The listing builds one solid part. Answer for the finished solid, in the listing's coordinates (mm). A direction names the side the tool comes from. Coordinates: 2 decimals unless noted, no trailing zeros. Write each loop counter-clockwise with the first axis right and the second up, starting at its lowest first coordinate (ties: lowest second). Pieces come first, ordered by that corner, then holes.
from build123d import *

# Parameters (mm, degrees)
SKETCH_1_R      = 2.5
SKETCH_1_R_2    = 4.5
SKETCH_1_R_3    = 3
SKETCH_1_R_4    = 1.5
EXTRUDE_1_DEPTH = 2.5


with BuildPart() as part:
    # Эскиз1 → Бобышка-Вытянуть1 (new, symmetric)
    # profile 1 of 7: a face of its own
    with BuildSketch(Plane.XY):
        with BuildLine():
            ThreePointArc((-0.9, -4.409081537), (-4.5, 0), (-0.9, 4.409081537))
            Line((-0.9, 4.409081537), (-10.5, 2.449489743))
            ThreePointArc((-10.5, 2.449489743), (-8.41886117, 1.936491673), (-7.5, 0))
            ThreePointArc((-7.5, 0), (-8.41886117, -1.936491673), (-10.5, -2.449489743))
            Line((-10.5, -2.449489743), (-0.9, -4.409081537))
        make_face()
    # profile 2 of 7: a face of its own
    with BuildSketch(Plane.XY):
        with Locations((-10, 0)):
            Circle(SKETCH_1_R)
    # profile 3 of 7: a face of its own
    with BuildSketch(Plane.XY):
        Circle(SKETCH_1_R_2)
        Circle(SKETCH_1_R, mode=Mode.SUBTRACT)
    # profile 4 of 7: a face of its own
    with BuildSketch(Plane.XY):
        with BuildLine():
            Line((12.375, 2.976470225), (0.5625, 4.464705337))
            ThreePointArc((0.5625, 4.464705337), (3.375, 2.976470225), (4.5, 0))
            ThreePointArc((4.5, 0), (3.375, -2.976470225), (0.5625, -4.464705337))
            Line((0.5625, -4.464705337), (12.375, -2.976470225))
            ThreePointArc((12.375, -2.976470225), (9, 0), (12.375, 2.976470225))
        make_face()
    # profile 5 of 7: a face of its own
    with BuildSketch(Plane.XY):
        with Locations((12, 0)):
            Circle(SKETCH_1_R_3)
        with Locations((12, 0)):
            Circle(SKETCH_1_R_4, mode=Mode.SUBTRACT)
    # profile 6 of 7: a face of its own
    with BuildSketch(Plane.XY):
        with BuildLine():
            Line((-1.5, -2), (-1.5, 2))
            ThreePointArc((-1.5, 2), (-2.5, 0), (-1.5, -2))
        make_face()
    # profile 7 of 7: a face of its own
    with BuildSketch(Plane.XY):
        with BuildLine():
            ThreePointArc((2.5, 0), (2.236067977, 1.118033989), (1.5, 2))
            Line((1.5, 2), (1.5, -2))
            ThreePointArc((1.5, -2), (2.236067977, -1.118033989), (2.5, 0))
        make_face()
    extrude(amount=EXTRUDE_1_DEPTH, both=True)


solid = part.part
1. Find the intervals of material crossed by L1, parallel to X at y = -1, z = -1.9; L2, parallel to Y at x = 12, z = 0.9; L3, parallel to X at y = 2.25, z = -1.1, in increasing order.
Results found:
L1: x = -12.29 to -1.5, 1.5 to 10.88, 13.12 to 14.83
L2: y = -3.02 to -1.5, 1.5 to 3.02
L3: x = -11.09 to -1.09, 1.09 to 13.98
2. Section D-D on x = 8.75 is taken. Give the vertices of the cut face in (y, z).
Results found:
outline: (-3.43, -2.5) - (3.43, -2.5) - (3.43, 2.5) - (-3.43, 2.5) - close
3. A tool of negligible diameter and unlimited length cuts with its end or side. For faces 1 (the flat face through (-5.767, -3.416, 0.035)), 2 (the cylindrical face through (0, 2.5, 0)), from which of +Z, -Z, +X, -X, +Y, -Y can it reach the whole face along a straight path? Write none if from no direction.
Results found:
face 1: +Z, -Z, -X, -Y
face 2: +Z, -Z
4. Flat-ended cylindrical pins translate along their axes: P1, Ø1.5, axis at x = -2, z = 0, coming from the +Y side; P2, Ø2, axis at y = 3.5, z = 0.5, coming from the +X side. Find the tip coordinate at first contact, or state that the pin passes through.
Results found:
P1: stops at y = 4.34
P2: stops at x = 13.66
5. Section A-A on y = 0 is taken. Give the vertices of the cut face in (x, z), then the cut area to 4 significant figures.
Results found:
outline: (-12.5, -2.5) - (-1.5, -2.5) - (-1.5, 2.5) - (-12.5, 2.5) - close; (1.5, -2.5) - (10.5, -2.5) - (10.5, 2.5) - (1.5, 2.5) - close; (13.5, -2.5) - (15, -2.5) - (15, 2.5) - (13.5, 2.5) - close
area: 107.5 mm2
6. For a pull along Y with two mould halves and no side action, classify faces 3 (the flat face through (1.5, 0, 0)), 4 (the cylindrical face through (0, -2.5, 0)), 5 (the flat face through (6.39, -3.73, 0.04)), 6 (the flat face through (-5.633, 3.443, 0.035)) as pulls with the +Y half, pulls with the -Y half, needs draft (parallel to the pull), parting line crosses it, or undercut.
Results found:
face 3: undercut
face 4: undercut
face 5: pulls with the -Y half
face 6: pulls with the +Y half
7. Section C-C on x = 12.75 is taken. Give the vertices of the cut face in (y, z), then the cut area to 3 significant figures.
Results found:
outline: (-2.9, -2.5) - (-1.3, -2.5) - (-1.3, 2.5) - (-2.9, 2.5) - close; (1.3, -2.5) - (2.9, -2.5) - (2.9, 2.5) - (1.3, 2.5) - close
area: 16.1 mm2
8. Section B-B on z = -1.05 is taken. Give the vertices of the cut face in (x, y) (1 decimal), then the cut area to 3 significant figures.
Results found:
outline: (-10.5, -2.4) - (-0.9, -4.4) arc R4.5 ccw to (0.6, -4.5) - (12.4, -3) arc R3 ccw to (12.4, 3) - (0.6, 4.5) arc R4.5 ccw to (-0.9, 4.4) - (-10.5, 2.4) arc R2.5 ccw to start; hole (-1.5, -2) arc R2.5 ccw to (1.5, -2) - (1.5, 2) arc R2.5 ccw to (-1.5, 2) - close; hole circle Ø3 at (12, 0)
area: 165 mm2
